Here's how the part is built. I have some questions about the finished solid (model axes, mm). Face numbers are marked on the shaded views. Round coordinates to 2 decimals unless told otherwise and drop trailing zeros. Write each loop counter-clockwise with the first axis right and the second up, starting at its lowest first coordinate (ties: lowest second). Pieces come first, ordered by that corner, then holes. Notation, with made-up numbers: (-3.5, 61) -> (9.5, 61) arc R22 cw to (9.5, 86) -> close; hole circle Ø10 at (63, 44.5). An arc over 180 degrees is marked (long way). Answer in a Markdown table with one row per item.
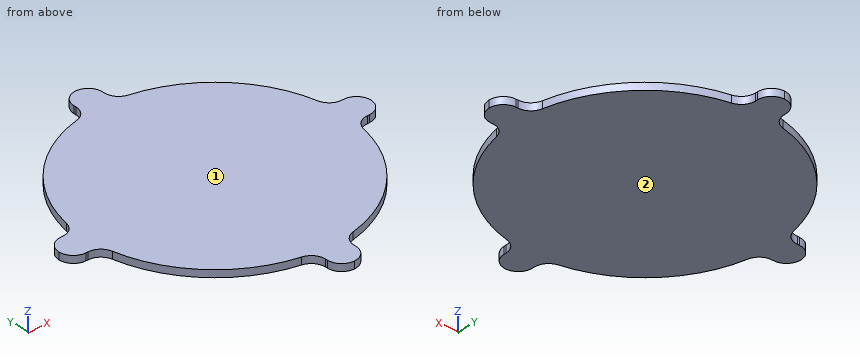
from build123d import *

# Parameters (mm, degrees)
F1_DEPTH = 25.4
F2_R     = 50.79999


# Not quite as in the source:
# - a fillet or chamfer is up to 0.001 mm smaller than in the source, because OpenCascade refuses the exact size


with BuildPart() as f1:
    # F0 (on Top) → F1 (new body)
    with BuildSketch(Plane.XY):
        with BuildLine():
            Line((-50.8, 555.969013028), (-50.8, 454.369013028))
            ThreePointArc((-50.8, 454.369013028), (-323.2892203585, 323.2892203585), (-454.369013028, 50.8))
            Line((-454.369013028, 50.8), (-555.969013028, 50.8))
            Line((-555.969013028, 50.8), (-555.969013028, -50.8))
            Line((-555.969013028, -50.8), (-454.369013028, -50.8))
            ThreePointArc((-454.369013028, -50.8), (-323.2892203585, -323.2892203585), (-50.8, -454.369013028))
            Line((-50.8, -454.369013028), (-50.8, -555.969013028))
            Line((-50.8, -555.969013028), (50.8, -555.969013028))
            Line((50.8, -555.969013028), (50.8, -454.369013028))
            ThreePointArc((50.8, -454.369013028), (323.2892203585, -323.2892203585), (454.369013028, -50.8))
            Line((454.369013028, -50.8), (555.969013028, -50.8))
            Line((555.969013028, -50.8), (555.969013028, 50.8))
            Line((555.969013028, 50.8), (454.369013028, 50.8))
            ThreePointArc((454.369013028, 50.8), (323.2892203585, 323.2892203585), (50.8, 454.369013028))
            Line((50.8, 454.369013028), (50.8, 555.969013028))
            Line((50.8, 555.969013028), (-50.8, 555.969013028))
        make_face()
    extrude(amount=F1_DEPTH)

    # F2 (radius 50.8 in the source; OpenCascade refuses exactly that, so slightly less here)
    f2_edges = [f1.edges().sort_by_distance(p)[0] for p in [
        (50.8, -555.969013, 12.7),
        (-50.8, -555.969013, 12.7),
        (555.969013, -50.8, 12.7),
        (555.969013, 50.8, 12.7),
        (50.8, 555.969013, 12.7),
        (-50.8, 555.969013, 12.7),
        (-555.969013, 50.8, 12.7),
        (-555.969013, -50.8, 12.7),
        (50.8, -454.369013, 12.7),
        (454.369013, -50.8, 12.7),
        (454.369013, 50.8, 12.7),
        (50.8, 454.369013, 12.7),
        (-50.8, 454.369013, 12.7),
        (-454.369013, 50.8, 12.7),
        (-454.369013, -50.8, 12.7),
        (-50.8, -454.369013, 12.7),
    ]]
    fillet(f2_edges, radius=F2_R)


solid = f1.part
1) I want a section at B-B, the plane x = 417. List the corners of the cut face in (y, z) for me, and give its area (3 significant figures).
Response:
| item | result |
|---|---|
| outline | (-187.46, 0) -> (187.46, 0) -> (187.46, 25.4) -> (-187.46, 25.4) -> close |
| area | 9,520 mm^2 |
2) For pin 1 (2 mm diameter, centred on y = -500, z = 10, fed in from +X); pin 2 (8 mm diameter, centred on x = 502, z = 16, fed in from -Y); pin 3 (4 mm diameter, centred on y = 238, z = 20, fed in from -X), each with a flat end and sliding along its axis, tell me the tip position at first contact or that it passes through.
Response:
| item | result |
|---|---|
| pin 1 | stops at x = 50.8 |
| pin 2 | stops at y = -50.8 |
| pin 3 | stops at x = -391.58 |
3) I need wall thicknesses on line 1 (X direction, y = 502, z = 18); line 2 (Y direction, x = 365, z = 18.75); line 3 (Y direction, x = -352, z = 22.25). Which ranges of each line are inside material? Lowest first, please. Write a range as [from, to].
Response:
| item | result |
|---|---|
| line 1 | x = [-50.8, 50.8] |
| line 2 | y = [-275.33, 275.33] |
| line 3 | y = [-291.77, 291.77] |
4) We'd pull the mould along Z, two halves only. Please class the marked faces 1 and 2: +Z half, -Z half, draft (parallel to the pull), parting line (faces both ways), or undercut.
Response:
| item | result |
|---|---|
| face 1 | +Z half |
| face 2 | -Z half |
5) I want a section at C-C, the plane y = -120. List the corners of the cut face in (x, z) for me.
Response:
| item | result |
|---|---|
| outline | (-441.17, 0) -> (441.17, 0) -> (441.17, 25.4) -> (-441.17, 25.4) -> close |
